For this review, take the finished solid that the model builds, in its own axes (mm). Face numbers are marked on the shaded views. A direction names the side the tool comes from. Coordinates: 2 decimals unless noted, no trailing zeros. Write each loop counter-clockwise with the first axis right and the second up, starting at its lowest first coordinate (ties: lowest second). Pieces come first, ordered by that corner, then holes.
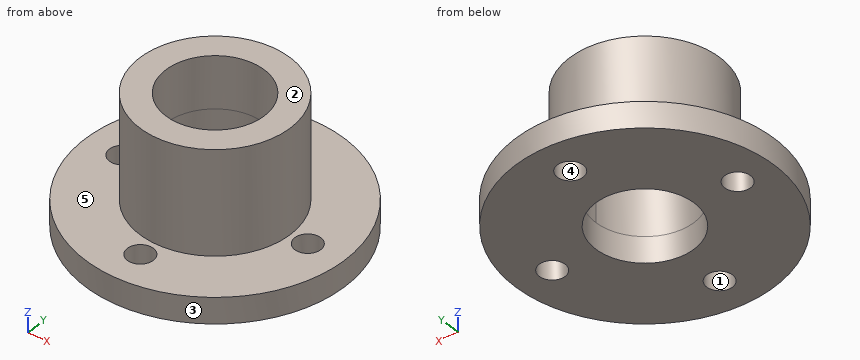
```python
from build123d import *
from build123d.topology import SkipClean

# Parameters (mm, degrees)
SKETCH1_R           = 25
BOSS_EXTRUDE1_DEPTH = 5
SKETCH2_R           = 14.5
SKETCH2_R_2         = 9.5
BOSS_EXTRUDE2_DEPTH = 20
SKETCH3_R           = 9.5
CUT_EXTRUDE1_DEPTH  = 15
SKETCH4_R           = 2.5
CUT_EXTRUDE2_DEPTH  = 10


with BuildPart() as part:
    # Sketch1 → Boss-Extrude1 (new body)
    with BuildSketch(Plane.XY):
        Circle(SKETCH1_R)
    extrude(amount=BOSS_EXTRUDE1_DEPTH)

    # Sketch2 → Boss-Extrude2 (add)
    with BuildSketch(Plane.XY.offset(5)):
        Circle(SKETCH2_R)
        Circle(SKETCH2_R_2, mode=Mode.SUBTRACT)
    extrude(amount=BOSS_EXTRUDE2_DEPTH)

    # Sketch3 → Cut-Extrude1 (cut)
    with SkipClean():  # the faces are left unmerged after this step: merging them gives an invalid solid
        with BuildSketch(Plane(origin=(0, 0, 0), x_dir=(-1, 0, 0), z_dir=(0, 0, -1))):
            Circle(SKETCH3_R)
        extrude(amount=-CUT_EXTRUDE1_DEPTH, mode=Mode.SUBTRACT)
    add(part.part.scale(1), mode=Mode.REPLACE)  # the faces are merged on a copy

    # Sketch4 → Cut-Extrude2 (cut)
    with BuildSketch(Plane(origin=(0, 0, 0), x_dir=(-1, 0, 0), z_dir=(0, 0, -1))):
        with Locations((0, 18)):
            Circle(SKETCH4_R)
        with Locations((18, 0)):
            Circle(SKETCH4_R)
        with Locations((0, -18)):
            Circle(SKETCH4_R)
        with Locations((-18, 0)):
            Circle(SKETCH4_R)
    extrude(amount=-CUT_EXTRUDE2_DEPTH, mode=Mode.SUBTRACT)


solid = part.part
```
Q1. Add section B-B (y = -18). State the section outline as (x, z) points.
Ans:
outline: (-17.35, 0) - (-2.5, 0) - (-2.5, 5) - (-17.35, 5) - close; (2.5, 0) - (17.35, 0) - (17.35, 5) - (2.5, 5) - close
Q2. Add section D-D (z = 2.25). State the section outline as (x, y) points, then the cut area to 3 significant figures.
Ans:
outline: circle Ø50 at (0, 0); hole circle Ø5 at (-18, 0); hole circle Ø19 at (0, 0); hole circle Ø5 at (0, -18); hole circle Ø5 at (0, 18); hole circle Ø5 at (18, 0)
area: 1,600 mm2
Q3. Add section C-C (x = 7.5). State the section outline as (y, z) points.
Ans:
outline: (-23.85, 0) - (-5.83, 0) - (-5.83, 25) - (-12.41, 25) - (-12.41, 5) - (-23.85, 5) - close; (5.83, 0) - (23.85, 0) - (23.85, 5) - (12.41, 5) - (12.41, 25) - (5.83, 25) - close
Q4. Add section A-A (x = 0). State the section outline as (y, z) points.
Ans:
outline: (-25, 0) - (-20.5, 0) - (-20.5, 5) - (-25, 5) - close; (-15.5, 0) - (-9.5, 0) - (-9.5, 25) - (-14.5, 25) - (-14.5, 5) - (-15.5, 5) - close; (9.5, 0) - (15.5, 0) - (15.5, 5) - (14.5, 5) - (14.5, 25) - (9.5, 25) - close; (20.5, 0) - (25, 0) - (25, 5) - (20.5, 5) - close
Q5. For probe 1 along Y at (x, z) = (0, 3.9); probe 2 along Y at (x, z) = (0, 17); probe 3 along Z at (x, y) = (-16, 4), list the stretches that pass through material, from the lowest coordinate up.
Ans:
probe 1: y = -25 to -20.5, -15.5 to -9.5, 9.5 to 15.5, 20.5 to 25
probe 2: y = -14.5 to -9.5, 9.5 to 14.5
probe 3: z = 0 to 5
Q6. Draft analysis for pull direction Y (two halves, no side actions). For the marked faces 1, 2 and 3, state which applies: +Y half, -Y half, draft (parallel to the pull), parting line (faces both ways), or undercut.
Ans:
face 1: undercut
face 2: draft
face 3: parting line
Q7. Tool access review of the marked faces 4 and 5: name each direction out of +Z, -Z, +X, -X, +Y, -Y from which nothing blocks a thin tool from reaching the whole face with its end or side.
Ans:
face 4: +Z, -Z
face 5: +Z
Q8. Clearance check with flat-ended pins moving along their axes: pin 1 Ø1.5 at (y, z) = (-4.5, 11.5) entering from -X; pin 2 Ø4 at (y, z) = (13.5, 5) entering from -X; pin 3 Ø6 at (x, z) = (10.5, 19.5) entering from -Y. State where each tip first meets the part, or that it passes through.
Ans:
pin 1: stops at x = -14.01
pin 2: stops at x = -22.2
pin 3: stops at y = -12.41
